Source: three-view drawing plus pictorial views. Frame: mm from the lowest corner of the part. A direction names the side the tool comes from. Give positions to 0.01 mm unless a question says otherwise; leave off trailing zeros. Write each loop counter-clockwise with the first axis right and the second up, starting at its lowest first coordinate (ties: lowest second). Pieces come first, ordered by that corner, then holes. Notation, with made-up numbers: (39.5, 64.25) -> (86.5, 64.25) arc R26 ccw to (86.5, 88.25) -> close; hole circle Ø2 at (76.5, 69). An arc over 180 degrees is marked (long way). Write item = value, one per line.
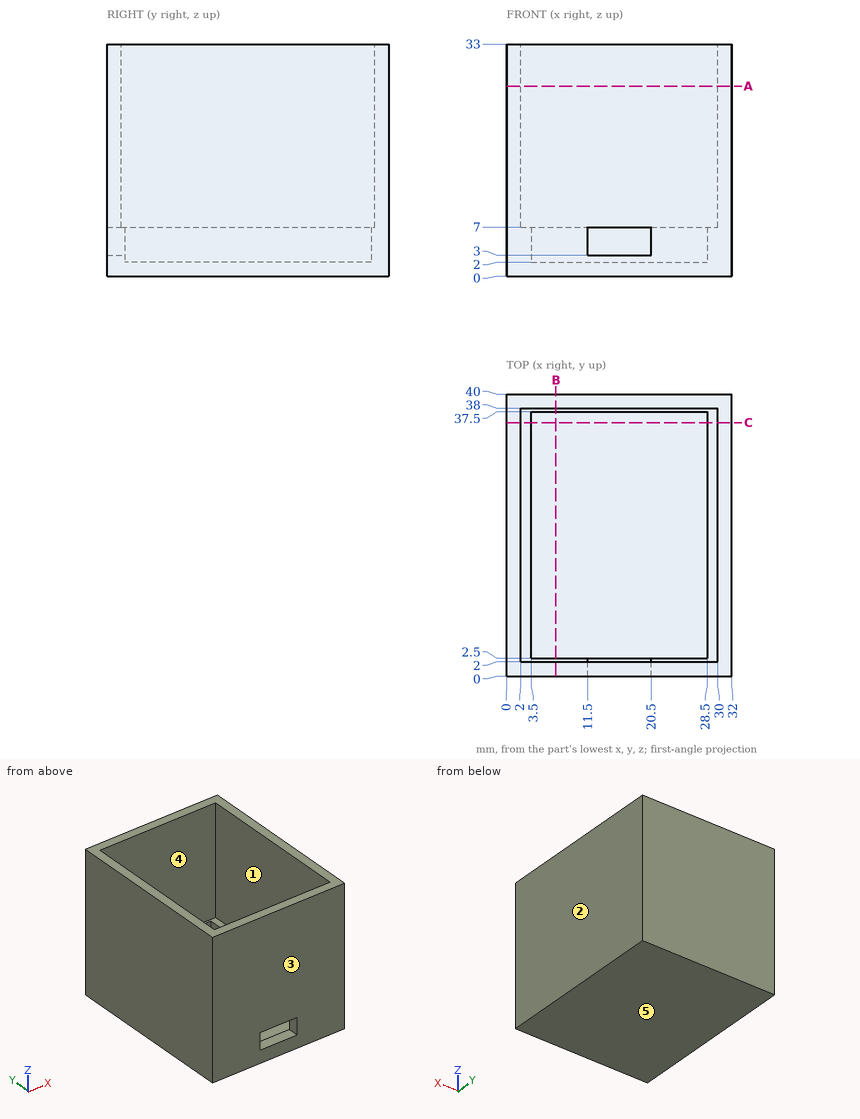
1) Material intervals for L1, parallel to Y at x = 16, z = 28; L2, parallel to X at y = 23, z = 21.5; L3, parallel to X at y = 30, z = 2.5, sorted ascending.
Computed:
L1 = 0 to 2, 38 to 40
L2 = 0 to 2, 30 to 32
L3 = 0 to 3.5, 28.5 to 32
2) Cut plane B-B (x = 7). Return the cut outline in (y, z).
Computed:
outline = (0, 0) -> (40, 0) -> (40, 33) -> (38, 33) -> (38, 7) -> (37.5, 7) -> (37.5, 2) -> (2.5, 2) -> (2.5, 7) -> (2, 7) -> (2, 33) -> (0, 33) -> close
3) Contact query for flat-ended pins moving along their axis: pin 1 (5.5 mm diameter, centred on x = 21, z = 4, fed in from -Y); pin 2 (12.5 mm diameter, centred on x = 19, y = 15, fed in from +Z). Output: stop coordinate, or through.
Computed:
pin_1 = 0
pin_2 = 2
4) Cut plane A-A (z = 27). Return the cut outline in (x, y), then the cut area to 3 significant figures.
Computed:
outline = (0, 0) -> (32, 0) -> (32, 40) -> (0, 40) -> close; hole (2, 2) -> (30, 2) -> (30, 38) -> (2, 38) -> close
area = 272 mm²
5) Draft query along Y for the marked faces 1, 2 and 3. Return one class per face: pulls with the +Y half, pulls with the -Y half, needs draft (parallel to the pull), parting line crosses it, or undercut.
Computed:
face_1 = undercut
face_2 = needs draft
face_3 = pulls with the -Y half
6) Cut plane C-C (y = 36). Return the cut outline in (x, z), then the cut area to 3 significant figures.
Computed:
outline = (0, 0) -> (32, 0) -> (32, 33) -> (30, 33) -> (30, 7) -> (28.5, 7) -> (28.5, 2) -> (3.5, 2) -> (3.5, 7) -> (2, 7) -> (2, 33) -> (0, 33) -> close
area = 203 mm²
7) Access query for the marked faces 4 and 5. Directions: +Z, -Z, +X, -X, +Y, -Y. A direction counts if a zero-diameter tool reaches every point of the face in a straight line with its end or side. Return the directions, or none.
Computed:
face_4 = +Z
face_5 = -Z, +X, -X, +Y, -Y
